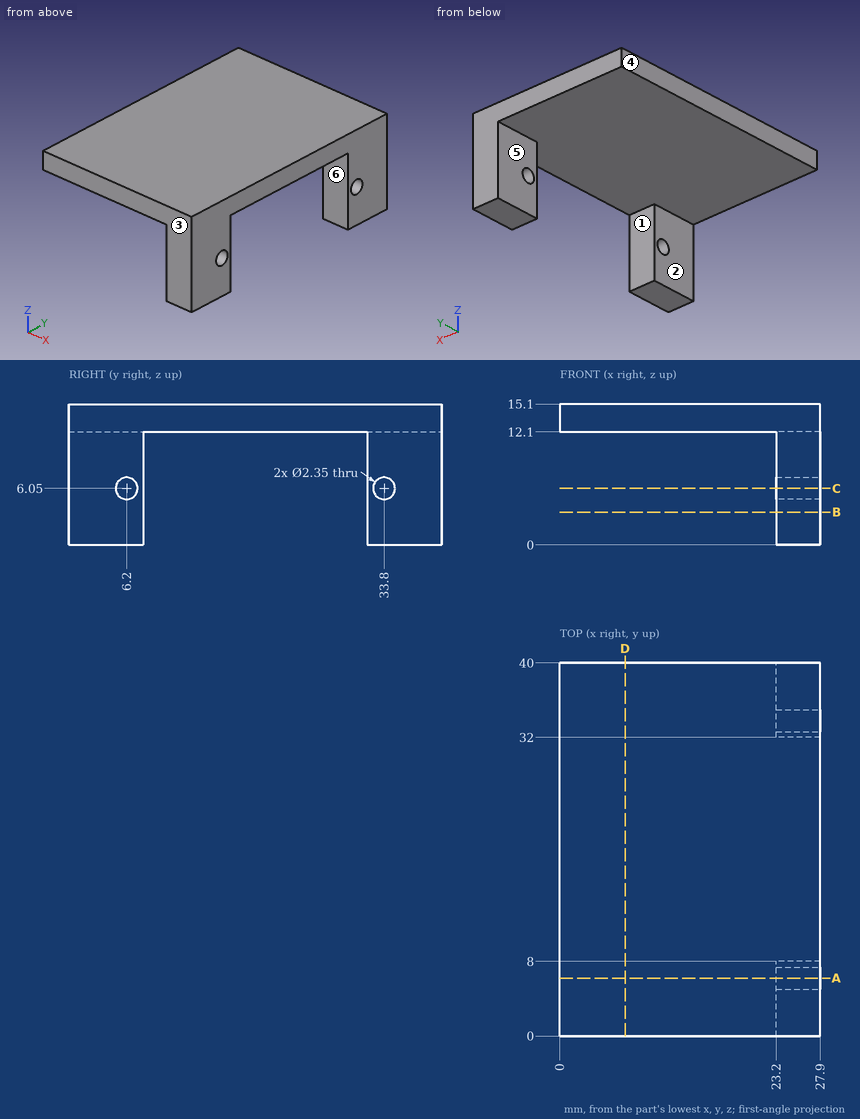
Could you check a few things on this drawing? It's one solid part, dimensions in mm from its lowest x, y, z. A direction names the side the tool comes from. Give positions to 0.01 mm unless a question says otherwise; leave off trailing zeros. Order: outer loops, then holes, each group sorted by start corner. A loop starts at its lowest first (then second) coordinate and runs counter-clockwise, first axis right, second up. Notation, with made-up numbers: (76, 55.5) -> (116, 55.5) arc R11 cw to (116, 61.5) -> close; hole circle Ø6 at (-6, 71). An arc over 180 degrees is marked (long way). Use CSV: the item, a comma, the result in double quotes. Start each with the question number.
Item 1: On a 3-axis mill with a long thin cutter (end or side, diameter ignored), from which of +Z, -Z, +X, -X, +Y, -Y can I reach the whole of each face in a straight line? I mean the marked faces 4, 5 and 6. Say none if no direction works.
Item 2: Thinking about a two-plate mould opening in Y: for the marked faces 1, 2 and 3, which applies, pulls with the +Y half, pulls with the -Y half, needs draft (parallel to the pull), parting line crosses it, or undercut?
Item 3: Suppose I cut it at D-D (x = 7). List the corners of the cut face in (y, z) for me, and give its area (3 significant figures).
Item 4: If I drill on probe 1 along Y at (x, z) = (26.5, 6.05) (3 decimals); probe 2 along Y at (x, z) = (26, 7); probe 3 along Z at (x, y) = (7, 38.5), over which ranges is the centre line in solid material (lowest first)? Write a range as [from, to].
Item 5: I'm going to push flat-ended pins straight in: P1, Ø9, axis at y = 36.5, z = 3.5, coming from the -X side; P2, Ø8.5, axis at x = 18.5, y = 28, coming from the -Z side. Where does each tip first touch, or does it pass through?
Item 6: Suppose I cut it at A-A (y = 6.2). List the corners of the cut face in (x, z) for me (3 decimals), and give its area (3 significant figures).
Item 7: Suppose I cut it at C-C (z = 6.05). List the corners of the cut face in (x, y) for me (3 decimals).
Item 8: Suppose I cut it at B-B (z = 3.5). List the corners of the cut face in (x, y) for me.
Answer block:
1,face 4,"+Z, -Z, -X, +Y, -Y"
1,face 5,"-Z, -X, +Y, -Y"
1,face 6,"-Z, +X, -X"
2,face 1,"undercut"
2,face 2,"needs draft"
2,face 3,"pulls with the -Y half"
3,outline,"(0, 12.1) -> (40, 12.1) -> (40, 15.1) -> (0, 15.1) -> close"
3,area,"120 mm^2"
4,probe 1,"y = [0, 5.025], [7.375, 8], [32, 32.625], [34.975, 40]"
4,probe 2,"y = [0, 5.51], [6.89, 8], [32, 33.11], [34.49, 40]"
4,probe 3,"z = [12.1, 15.1]"
5,P1,"stops at x = 23.2"
5,P2,"stops at z = 12.1"
6,outline,"(0, 12.1) -> (23.2, 12.1) -> (23.2, 7.225) -> (27.9, 7.225) -> (27.9, 15.1) -> (0, 15.1) -> close; (23.2, 0) -> (27.9, 0) -> (27.9, 4.875) -> (23.2, 4.875) -> close"
6,area,"130 mm^2"
7,outline,"(23.2, 0) -> (27.9, 0) -> (27.9, 5.025) -> (23.2, 5.025) -> close; (23.2, 7.375) -> (27.9, 7.375) -> (27.9, 8) -> (23.2, 8) -> close; (23.2, 32) -> (27.9, 32) -> (27.9, 32.625) -> (23.2, 32.625) -> close; (23.2, 34.975) -> (27.9, 34.975) -> (27.9, 40) -> (23.2, 40) -> close"
8,outline,"(23.2, 0) -> (27.9, 0) -> (27.9, 8) -> (23.2, 8) -> close; (23.2, 32) -> (27.9, 32) -> (27.9, 40) -> (23.2, 40) -> close"
